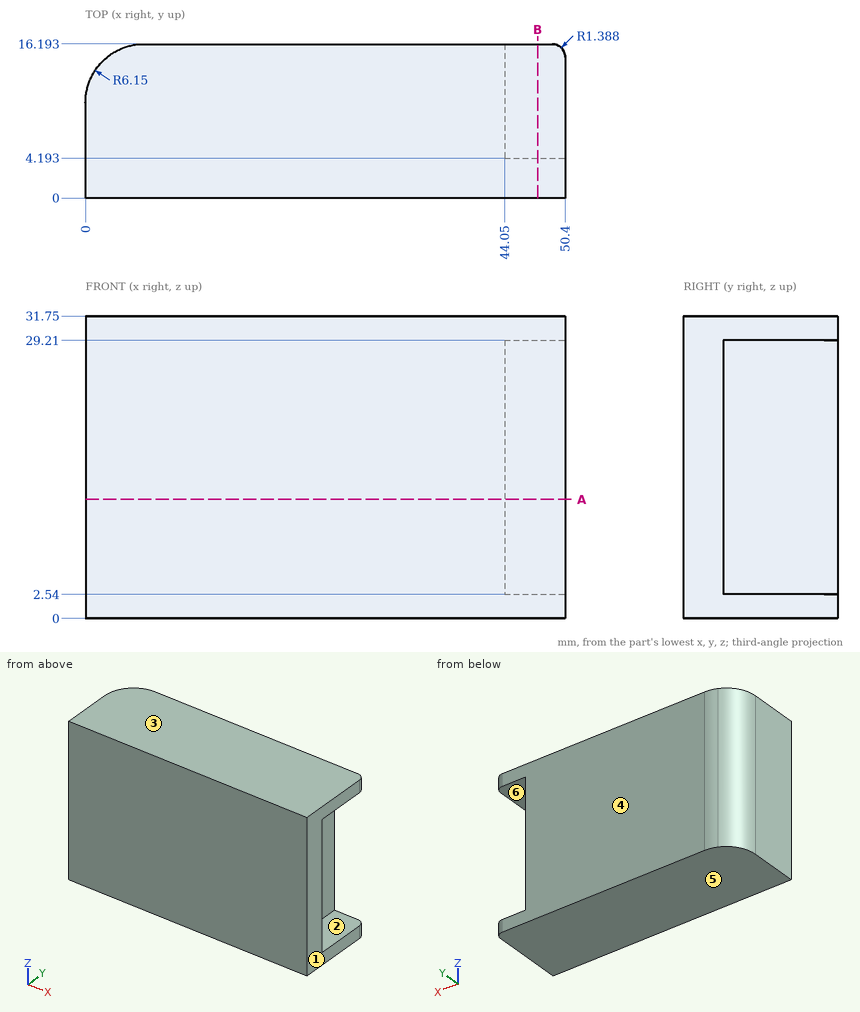
Verification items for this drawing (mm, ordinates from the low corner). A direction names the side the tool comes from. Coordinates: 2 decimals unless noted, no trailing zeros. Loops run counter-clockwise (first coordinate to the right, second up) from the corner with the lowest first, then second, coordinate; pieces in that order, holes last. Notation, with made-up numbers: (54.5, 80) - (70.5, 80) arc R20 cw to (70.5, 116) - close; hole circle Ø9 at (-14.75, 18.25). An arc over 180 degrees is marked (long way). One line per item, written item: value. Start each with the question number.
(1) Material ranges on line 1 (Z direction, x = 45, y = 8.5); line 2 (Y direction, x = 45, z = 6.5); line 3 (X direction, y = 8, z = 24), recorded low to high. Write a range as [from, to].
(2) Depth check by flat-ended pin: P1, Ø3.5, axis at y = 13, z = 11.5, coming from the +X side; P2, Ø3, axis at x = 47.5, z = 16, coming from the +Y side. Enter the tip coordinate at first touch or a pass-through.
(3) Cross-section at A-A on z = 12.5. Enter the section's corners in (x, y), plus the area to 3 significant figures.
(4) Tool access check on the marked faces 1 and 2. Record the directions out of +Z, -Z, +X, -X, +Y, -Y that give a thin tool (end or side, any length) a straight path to the whole face; none if there is none.
(5) Mould release check, pull along Z, two halves, no side actions. Record for the marked faces 3, 4, 5 and 6: released by +Z, released by -Z, zero draft, split by the parting line, or undercut.
(6) Cross-section at B-B on x = 47.5. Enter the section's corners in (y, z).
Results below:
1. line 1: z = [0, 2.54], [29.21, 31.75]
1. line 2: y = [0, 4.19]
1. line 3: x = [0, 44.05]
2. P1: stops at x = 44.05
2. P2: stops at y = 4.19
3. outline: (0, 0) - (50.4, 0) - (50.4, 4.19) - (44.05, 4.19) - (44.05, 16.19) - (6.15, 16.19) arc R6.15 ccw to (0, 10.04) - close
3. area: 732 mm2
4. face 1: +Z, -Z, +X, +Y, -Y
4. face 2: +X, +Y
5. face 3: released by +Z
5. face 4: zero draft
5. face 5: released by -Z
5. face 6: undercut
6. outline: (0, 0) - (16.19, 0) - (16.19, 2.54) - (4.19, 2.54) - (4.19, 29.21) - (16.19, 29.21) - (16.19, 31.75) - (0, 31.75) - close
